For this review, take the finished solid that the model builds, in its own axes (mm). A direction names the side the tool comes from. Coordinates: 2 decimals unless noted, no trailing zeros. Loops run counter-clockwise (first coordinate to the right, second up) from the corner with the lowest first, then second, coordinate; pieces in that order, holes last. Notation, with made-up numbers: (-5.5, 40) -> (41.5, 40) arc R18 cw to (41.5, 71) -> close; hole circle Ø10 at (16, -17). An arc over 180 degrees is marked (long way). Answer in a Markdown table with one row per item.
from build123d import *

# Parameters (mm, degrees)
F0_W      = 25
F0_H      = 20
F1_DEPTH  = 32
F2_R      = 1.25
F2_R_2    = 1.5
F3_DEPTH  = 19
F5_DEPTH  = 10
F7_DEPTH  = 11.5
F8_R      = 3
F8_R_2    = 1.5
F9_DEPTH  = 20.001
F10_R     = 1.25
F10_R_2   = 0.75
F11_DEPTH = 5
F12_R     = 2
F13_DEPTH = 3.5
F14_W     = 20
F14_H     = 5
F15_DEPTH = 25
F16_W     = 15
F16_H     = 20
F16_R     = 1.5875
F17_DEPTH = 2


with BuildPart() as f1:
    # F0 (on Top) → F1 (new body)
    with BuildSketch(Plane.XY):
        with Locations((12.5, 10)):
            Rectangle(F0_W, F0_H)
    extrude(amount=F1_DEPTH)

    # F2 (on face) → F3 (join)
    with BuildSketch(Plane.XZ):
        with BuildLine():
            Line((17.5, 30.5), (7.5, 30.5))
            ThreePointArc((7.5, 30.5), (4.671573, 29.328427), (3.5, 26.5))
            Line((3.5, 26.5), (3.5, 16.5))
            ThreePointArc((3.5, 16.5), (4.671573, 13.671573), (7.5, 12.5))
            Line((7.5, 12.5), (17.5, 12.5))
            ThreePointArc((17.5, 12.5), (20.328427, 13.671573), (21.5, 16.5))
            Line((21.5, 16.5), (21.5, 26.5))
            ThreePointArc((21.5, 26.5), (20.328427, 29.328427), (17.5, 30.5))
        make_face()
        with Locations((7.5, 17)):
            Circle(F2_R, mode=Mode.SUBTRACT)
        with Locations((17.5, 17)):
            Circle(F2_R, mode=Mode.SUBTRACT)
        with Locations((7.5, 21.5)):
            Circle(F2_R, mode=Mode.SUBTRACT)
        with Locations((7.5, 26)):
            Circle(F2_R, mode=Mode.SUBTRACT)
        with Locations((12.5, 26)):
            Circle(F2_R_2, mode=Mode.SUBTRACT)
        with Locations((17.5, 21.5)):
            Circle(F2_R, mode=Mode.SUBTRACT)
        with Locations((17.5, 26)):
            Circle(F2_R, mode=Mode.SUBTRACT)
    extrude(amount=F3_DEPTH)

    # F4 (on face) → F5 (cut)
    with BuildSketch(Plane(origin=(0, 20, 0), x_dir=(-1, 0, 0), z_dir=(0, 1, 0))):
        with BuildLine():
            Line((-7.5, 30.5), (-17.5, 30.5))
            ThreePointArc((-17.5, 30.5), (-20.328427, 29.328427), (-21.5, 26.5))
            Line((-21.5, 26.5), (-21.5, 16.5))
            ThreePointArc((-21.5, 16.5), (-20.328427, 13.671573), (-17.5, 12.5))
            Line((-17.5, 12.5), (-7.5, 12.5))
            ThreePointArc((-7.5, 12.5), (-4.671573, 13.671573), (-3.5, 16.5))
            Line((-3.5, 16.5), (-3.5, 26.5))
            ThreePointArc((-3.5, 26.5), (-4.671573, 29.328427), (-7.5, 30.5))
        make_face()
    extrude(amount=-F5_DEPTH, mode=Mode.SUBTRACT)

    # F6 (on face) → F7 (join)
    with BuildSketch(Plane.XZ):
        with BuildLine():
            Line((15, 12.5), (10, 12.5))
            Line((10, 12.5), (10.445252, 8.937983))
            ThreePointArc((10.445252, 8.937983), (10.61049, 8.625161), (10.941391, 8.5))
            Line((10.941391, 8.5), (14.058609, 8.5))
            ThreePointArc((14.058609, 8.5), (14.38951, 8.625161), (14.554748, 8.937983))
            Line((14.554748, 8.937983), (15, 12.5))
        make_face()
    extrude(amount=F7_DEPTH)

    # F8 (on face) → F9 (cut, through all)
    with BuildSketch(Plane.XZ):
        with Locations((12.5, 26)):
            Circle(F8_R)
        with Locations((7.5, 26)):
            Circle(F8_R_2)
        with Locations((7.5, 21.5)):
            Circle(F8_R_2)
        with Locations((7.5, 17)):
            Circle(F8_R_2)
        with Locations((17.5, 26)):
            Circle(F8_R_2)
        with Locations((17.5, 21.5)):
            Circle(F8_R_2)
        with Locations((17.5, 17)):
            Circle(F8_R_2)
    extrude(amount=-F9_DEPTH, mode=Mode.SUBTRACT)

    # F10 (on face) → F11 (join)
    with BuildSketch(Plane.XZ):
        with Locations((7.5, 26)):
            Circle(F10_R)
        with Locations((7.5, 26)):
            Circle(F10_R_2, mode=Mode.SUBTRACT)
        with Locations((7.5, 21.5)):
            Circle(F10_R)
        with Locations((7.5, 21.5)):
            Circle(F10_R_2, mode=Mode.SUBTRACT)
        with Locations((7.5, 17)):
            Circle(F10_R)
        with Locations((7.5, 17)):
            Circle(F10_R_2, mode=Mode.SUBTRACT)
        with Locations((17.5, 26)):
            Circle(F10_R)
        with Locations((17.5, 26)):
            Circle(F10_R_2, mode=Mode.SUBTRACT)
        with Locations((17.5, 21.5)):
            Circle(F10_R)
        with Locations((17.5, 21.5)):
            Circle(F10_R_2, mode=Mode.SUBTRACT)
        with Locations((17.5, 17)):
            Circle(F10_R)
        with Locations((17.5, 17)):
            Circle(F10_R_2, mode=Mode.SUBTRACT)
    extrude(amount=F11_DEPTH)

    # F12 (on face) → F13 (cut, through all)
    with BuildSketch(Plane(origin=(0, 0, 0), x_dir=(0, -1, 0), z_dir=(-1, 0, 0))):
        with Locations((-15, 21)):
            Circle(F12_R)
    extrude(amount=-F13_DEPTH, mode=Mode.SUBTRACT)

    # F14 (on face) → F15 (cut)
    with BuildSketch(Plane(origin=(0, 0, 0), x_dir=(0, -1, 0), z_dir=(-1, 0, 0))):
        with Locations((-10, 2.5)):
            Rectangle(F14_W, F14_H)
    extrude(amount=-F15_DEPTH, mode=Mode.SUBTRACT)

    # F16 (on face) → F17 (join)
    with BuildSketch(Plane(origin=(0, 0, 5), x_dir=(1, 0, 0), z_dir=(0, 0, -1))):
        with Locations((32.5, -10)):
            Rectangle(F16_W, F16_H)
        with Locations((32.4125, -10)):
            Circle(F16_R, mode=Mode.SUBTRACT)
        with Locations((-7.5, -10)):
            Rectangle(F16_W, F16_H)
        with Locations((-7.4125, -10)):
            Circle(F16_R, mode=Mode.SUBTRACT)
    extrude(amount=-F17_DEPTH)


solid = f1.part
Item 1: Take a section at A-A, the plane y = 9. Count the separate pieces of the cut face and the enclosed holes in it, and give its area (3 significant figures).
Worked answers:
| item | result |
|---|---|
| separate pieces | 3 |
| enclosed holes | 7 |
| area | 654 mm² |
Item 2: Insertion check: pin 1 (5 mm diameter, centred on y = 2, z = 10, fed in from +X); pin 2 (9 mm diameter, centred on x = 8.5, z = 23, fed in from +Y); pin 3 (7.5 mm diameter, centred on x = 33.5, y = 9, fed in from +Z). Each pin has a flat end and moves straight along its axis. Give the tip position at first contact, or say it passes through.
Worked answers:
| item | result |
|---|---|
| pin 1 | x = 25 |
| pin 2 | y = 10 |
| pin 3 | z = 7 |
Item 3: Take a section at D-D, the plane x = -7.5. State the section outline as (y, z) points, and give its area (3 significant figures).
Worked answers:
| item | result |
|---|---|
| outline | (0, 5) -> (8.41, 5) -> (8.41, 7) -> (0, 7) -> close; (11.59, 5) -> (20, 5) -> (20, 7) -> (11.59, 7) -> close |
| area | 33.7 mm² |
Item 4: For L1, parallel to Z at x = 17.5, y = 2.75; L2, parallel to Z at x = 17.5, y = -13.75; L3, parallel to Z at x = 30, y = 9, list the stretches that pass through material, from the lowest coordinate up.
Worked answers:
| item | result |
|---|---|
| L1 | 5 to 15.5, 18.5 to 20, 23 to 24.5, 27.5 to 32 |
| L2 | 12.5 to 15.75, 18.25 to 20.25, 22.75 to 24.75, 27.25 to 30.5 |
| L3 | 5 to 7 |
Item 5: Take a section at C-C, the plane y = -15.5. State the section outline as (x, z) points, and give its area (3 significant figures).
Worked answers:
| item | result |
|---|---|
| outline | (3.5, 16.5) arc R4 ccw to (7.5, 12.5) -> (17.5, 12.5) arc R4 ccw to (21.5, 16.5) -> (21.5, 26.5) arc R4 ccw to (17.5, 30.5) -> (7.5, 30.5) arc R4 ccw to (3.5, 26.5) -> close; hole circle Ø2.5 at (7.5, 17); hole circle Ø2.5 at (7.5, 21.5); hole circle Ø2.5 at (7.5, 26); hole circle Ø3 at (12.5, 26); hole circle Ø2.5 at (17.5, 17); hole circle Ø2.5 at (17.5, 21.5); hole circle Ø2.5 at (17.5, 26) |
| area | 274 mm² |
Item 6: The part is to be moulded in two halves that separate along Y. For faces 5 (the flat face through (18, 0, 18)), 6 (the cylindrical face through (30.827, 9.93, 5.986)), 7 (the cylindrical face through (6.39, 4.93, 18.01)), 8 (the flat face through (16, 0, 11)), say which applies: +Y half, -Y half, draft (parallel to the pull), parting line (faces both ways), or undercut.
Worked answers:
| item | result |
|---|---|
| face 5 | +Y half |
| face 6 | undercut |
| face 7 | draft |
| face 8 | -Y half |
Item 7: For faces 1 (the flat face through (25, 10, 19)), 2 (the cylindrical face through (6.579, -11.902, 17.845)), 3 (the flat face through (10.22, -5.67, 10.74)), 4 (the cylindrical face through (4.703, 15.07, 13.641)), list the 3-axis set-ups (+Z, -Z, +X, -X, +Y, -Y) from which the entire face can be reached by the end or side of a thin tool; tool diameter is ignored.
Worked answers:
| item | result |
|---|---|
| face 1 | +Z, +X, +Y, -Y |
| face 2 | -Y |
| face 3 | -Z, -X, -Y |
| face 4 | +Y |
Item 8: Take a section at B-B, the plane x = 1. State the section outline as (y, z) points.
Worked answers:
| item | result |
|---|---|
| outline | (0, 5) -> (20, 5) -> (20, 32) -> (0, 32) -> close; hole circle Ø4 at (15, 21) |
